Geometry: final body of the model. Coordinates: model frame, mm. Face numbers are marked on the shaded views. Round coordinates to 2 decimals unless told otherwise and drop trailing zeros. Order: outer loops, then holes, each group sorted by start corner. A loop starts at its lowest first (then second) coordinate and runs counter-clockwise, first axis right, second up. Notation, with made-up numbers: (27, -20) -> (64, -20) arc R30 cw to (64, 15) -> close; hole circle Ø3 at (35.25, 16). An arc over 180 degrees is marked (long way). Put each result on its own line as item: value.
```python
from build123d import *

# Parameters (mm, degrees)
BOSS_EXTRUDE4_DEPTH = 6.1
BOSS_EXTRUDE5_START = 20
BOSS_EXTRUDE5_DEPTH = 20
SKETCH7_R           = 2.75
CUT_EXTRUDE1_DEPTH  = 109.516757445
SKETCH8_R           = 6
CUT_EXTRUDE2_DEPTH  = 20


with BuildPart() as part:
    # Sketch5 → Boss-Extrude4 (new body)
    with BuildSketch(Plane.XY):
        with BuildLine():
            Line((-89.802561211, 89.802561211), (-50.105122421, 129.5))
            Line((-50.105122421, 129.5), (50.105122421, 129.5))
            Line((50.105122421, 129.5), (89.802561211, 89.802561211))
            Line((89.802561211, 89.802561211), (98.994949366, 98.994949366))
            ThreePointArc((98.994949366, 98.994949366), (0, 140), (-98.994949366, 98.994949366))
            Line((-98.994949366, 98.994949366), (-89.802561211, 89.802561211))
        make_face()
    extrude(amount=-BOSS_EXTRUDE4_DEPTH)

    # Sketch6 → Boss-Extrude5 (add)
    with BuildSketch(Plane.XY.offset(BOSS_EXTRUDE5_START)):
        with BuildLine():
            Line((0, 129.5), (-53.195394538, 129.5))
            ThreePointArc((-53.195394538, 129.5), (0, 140), (53.195394538, 129.5))
            Line((53.195394538, 129.5), (0, 129.5))
        make_face()
    extrude(amount=-BOSS_EXTRUDE5_DEPTH)

    # Sketch7 → Cut-Extrude1 (cut, through all)
    with BuildSketch(Plane.XZ.offset(-129.5)):
        with Locations(Location((0, 10, 0), (0, 0, 270))):
            Circle(SKETCH7_R)
    extrude(amount=-CUT_EXTRUDE1_DEPTH, mode=Mode.SUBTRACT)

    # Sketch8 → Cut-Extrude2 (cut)
    with BuildSketch(Plane(origin=(0, 133.5, 0), x_dir=(-1, 0, 0), z_dir=(0, -1, 0))):
        with Locations(Location((0, -10, 0), (0, 0, 90))):
            Circle(SKETCH8_R)
    extrude(amount=-CUT_EXTRUDE2_DEPTH, mode=Mode.SUBTRACT)


solid = part.part
```
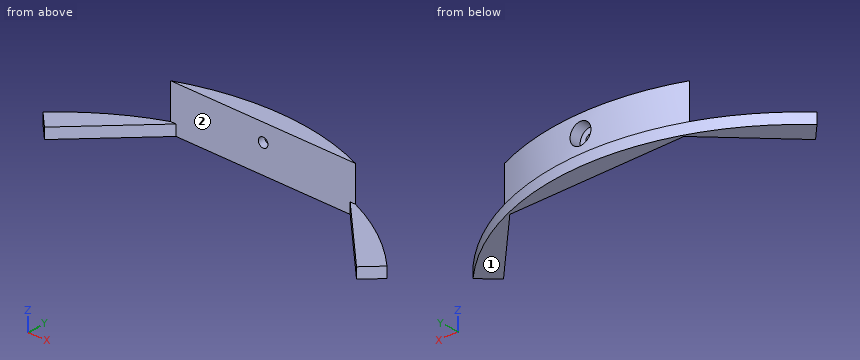
1. Material intervals for probe 1 along Z at (x, y) = (0, 138); probe 2 along X at (y, z) = (100, -3); probe 3 along Z at (x, y) = (2.5, 134), sorted ascending.
Ans:
probe 1: -6.1 to 4, 16 to 20
probe 2: -97.98 to -79.61, 79.61 to 97.98
probe 3: -6.1 to 4.55, 15.45 to 20
2. Contact query for flat-ended pins moving along their axis: P1, Ø12, axis at x = -32, z = 9.5, coming from the -Y side; P2, Ø12, axis at y = 131, z = -0.5, coming from the -X side; P3, Ø8, axis at x = 11, z = 8, coming from the +Y side. Output: stop coordinate, or through.
Ans:
P1: y = 129.5
P2: x = -63.05
P3: y = 139.82
3. Draft query along X for the marked faces 1 and 2. Return one class per face: +X half, -X half, draft (parallel to the pull), parting line (faces both ways), or undercut.
Ans:
face 1: draft
face 2: undercut
4. Cut plane B-B on z = 10. Return loops of the section in (x, y).
Ans:
outline: (-53.2, 129.5) -> (-2.75, 129.5) -> (-2.75, 133.5) -> (-6, 133.5) -> (-6, 139.87) arc R140 ccw to start; (2.75, 129.5) -> (53.2, 129.5) arc R140 ccw to (6, 139.87) -> (6, 133.5) -> (2.75, 133.5) -> close
5. Cut plane A-A on x = 0. Return loops of the section in (y, z).
Ans:
outline: (129.5, -6.1) -> (140, -6.1) -> (140, 4) -> (133.5, 4) -> (133.5, 7.25) -> (129.5, 7.25) -> close; (129.5, 12.75) -> (133.5, 12.75) -> (133.5, 16) -> (140, 16) -> (140, 20) -> (129.5, 20) -> close
6. Cut plane C-C on x = 86.5. Return loops of the section in (y, z).
Ans:
outline: (93.11, -6.1) -> (110.08, -6.1) -> (110.08, 0) -> (93.11, 0) -> close
7. Cut plane D-D on x = -41.5. Return loops of the section in (y, z), and give its area (3 significant figures).
Ans:
outline: (129.5, -6.1) -> (133.71, -6.1) -> (133.71, 20) -> (129.5, 20) -> close
area: 110 mm²
